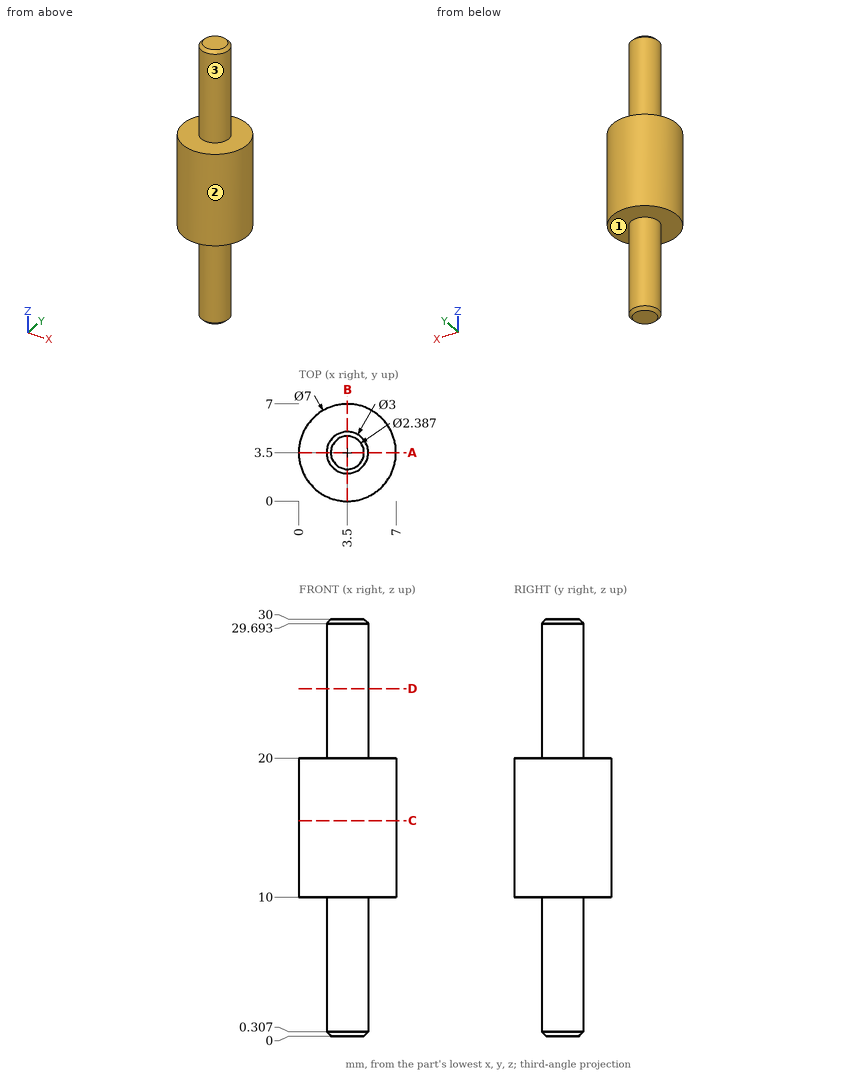
For this review, use the dimensioned drawing (mm, ordinates from the lowest corner) and the shaded views. A direction names the side the tool comes from. Round coordinates to 2 decimals unless told otherwise and drop trailing zeros. Order: outer loops, then holes, each group sorted by start corner. A loop starts at its lowest first (then second) coordinate and runs counter-clockwise, first axis right, second up. Notation, with made-up numbers: M 30.25,-24.75 L 42.25,-24.75 A22 cw 42.25,5.25 Z; hole C 67,71 d9. An arc over 180 degrees is marked long. Write each question's results on one line, items separated by ' | '. Start each with the question number.
1. Clearance check with a flat-ended pin moving along its axis: pin 1 Ø4 at (y, z) = (4.5, 27) entering from +X. State where the tip first meets the part, or that it passes through.
2. To check wall thickness, follow L1, parallel to Z at x = 1, y = 4.5; L2, parallel to X at y = 4.5, z = 12 (1 decimal); L3, parallel to X at y = 0.75, z = 16 (1 decimal). State the ranges of each line that lie inside material, in increasing order. Write a range as [from, to].
3. Add section D-D (z = 25). State the section outline as (x, y) points.
4. Add section A-A (y = 3.5). State the section outline as (x, z) points.
5. Add section C-C (z = 15.5). State the section outline as (x, y) points.
6. Tool access review of the marked faces 1, 2 and 3: name each direction out of +Z, -Z, +X, -X, +Y, -Y from which nothing blocks a thin tool from reaching the whole face with its end or side.
Output values:
1) pin 1: x = 5
2) L1: [10, 20] | L2: [0.1, 6.9] | L3: [1.3, 5.7]
3) outline: C 3.5,3.5 d3
4) outline: M 0,10 L 2,10 L 2,0.31 L 2.31,0 L 4.69,0 L 5,0.31 L 5,10 L 7,10 L 7,20 L 5,20 L 5,29.69 L 4.69,30 L 2.31,30 L 2,29.69 L 2,20 L 0,20 Z
5) outline: C 3.5,3.5 d7
6) face 1: -Z | face 2: +Z, -Z | face 3: +Z
